Can you work these out from the model? Positions are in its coordinate system, mm. Give positions to 0.01 mm unless a question says otherwise; leave off trailing zeros. Write each loop counter-clockwise with the first axis right and the second up, starting at its lowest first coordinate (ties: lowest second). Pieces come first, ordered by that corner, then holes. Notation, with made-up numbers: M 33,-9 L 59,-9 A26 ccw 59,21 Z; hole C -3,55.5 d6. An arc over 180 degrees is marked long. Answer as CSV lines item,"result". Start each with the question number.
```python
from build123d import *

# Parameters (mm, degrees)
BOSS_EXTRUDE1_DEPTH = 1.19
SKETCH2_R           = 3.97875
SKETCH2_R_2         = 3.98
CUT_EXTRUDE1_DEPTH  = 1.19


with BuildPart() as part:
    # Sketch1 → Boss-Extrude1 (new body)
    with BuildSketch(Plane(origin=(0, 0, 0), x_dir=(1, 0, 0), z_dir=(0, 1, 0))):
        Polygon((0, 0), (80, 0), (80, 20), (20, 20), (20, 80), (0, 80), align=None)
    extrude(amount=BOSS_EXTRUDE1_DEPTH)

    # Sketch2 → Cut-Extrude1 (cut)
    with BuildSketch(Plane(origin=(0, 1.19, 0), x_dir=(1, 0, 0), z_dir=(0, 1, 0))):
        with Locations((10, 61.34)):
            Circle(SKETCH2_R)
        with Locations((10, 35.94)):
            Circle(SKETCH2_R_2)
        with Locations((10, 10.54)):
            Circle(SKETCH2_R_2)
        with Locations((35.4, 10)):
            Circle(SKETCH2_R_2)
        with Locations((60.8, 10)):
            Circle(SKETCH2_R_2)
    extrude(amount=-CUT_EXTRUDE1_DEPTH, mode=Mode.SUBTRACT)


solid = part.part
```
1) I want a section at B-B, the plane x = 35.4. Please give me the cut outline in (y, z).
2) I want a section at D-D, the plane y = 1. Please give me the cut outline in (x, z).
3) Thinking about a two-plate mould opening in Z: for faces 1 (the flat face through (22, 0, -14)), 2 (the cylindrical face through (6.84, 0.6, -8.12)), 3 (the cylindrical face through (9.137, 0.603, -32.055)), which applies, released by +Z, released by -Z, zero draft, split by the parting line, or undercut?
4) I want a section at C-C, the plane x = 10. Please give me the cut outline in (y, z).
5) I need wall thicknesses on L1, parallel to Z at x = 10, y = 0.4; L2, parallel to X at y = 0.5, z = -35.5; L3, parallel to X at y = 1.05, z = -12.5. Which ranges of each line are inside material? Lowest first, please. Write a range as from..to.
6) I want a section at A-A, the plane z = -35.94. Please give me the cut outline in (x, y), then the cut area to 3 significant figures.
7) I'm going to push a flat-ended pin straight in: P1, Ø5, axis at x = 10, z = -10.54, coming from the -Y side. Where does the tip first touch, or does it pass through?
Values found:
1,outline,"M 0,-20 L 1.19,-20 L 1.19,-13.98 L 0,-13.98 Z; M 0,-6.02 L 1.19,-6.02 L 1.19,0 L 0,0 Z"
2,outline,"M 0,-80 L 20,-80 L 20,-20 L 80,-20 L 80,0 L 0,0 Z; hole C 10,-61.34 d7.96; hole C 10,-35.94 d7.96; hole C 10,-10.54 d7.96; hole C 35.4,-10 d7.96; hole C 60.8,-10 d7.96"
3,face 1,"zero draft"
3,face 2,"undercut"
3,face 3,"undercut"
4,outline,"M 0,-80 L 1.19,-80 L 1.19,-65.32 L 0,-65.32 Z; M 0,-57.36 L 1.19,-57.36 L 1.19,-39.92 L 0,-39.92 Z; M 0,-31.96 L 1.19,-31.96 L 1.19,-14.52 L 0,-14.52 Z; M 0,-6.56 L 1.19,-6.56 L 1.19,0 L 0,0 Z"
5,L1,"z = -80..-65.32, -57.36..-39.92, -31.96..-14.52, -6.56..0"
5,L2,"x = 0..6.04, 13.96..20"
5,L3,"x = 0..6.54, 13.46..32.3, 38.5..57.7, 63.9..80"
6,outline,"M 0,0 L 6.02,0 L 6.02,1.19 L 0,1.19 Z; M 13.98,0 L 20,0 L 20,1.19 L 13.98,1.19 Z"
6,area,"14.3 mm²"
7,P1,"passes through"
